Autodesk Inventor part; units mm, degrees
ref_plane "YZ Plane" through (0, 0, 0) normal (1, 0, 0) x (0, 1, 0)
ref_plane "XZ Plane" through (0, 0, 0) normal (0, 1, 0) x (-1, 0, 0)
ref_plane "XY Plane" through (0, 0, 0) normal (0, 0, 1) x (1, 0, 0)
sketch "Sketch1" plane through (0, 0, 0) normal (1, 0, 0) x (0, 1, 0)
  line L0 (-15, 42.5) -> (15, 42.5)
  line L1 (15, 42.5) -> (15, 37.5)
  line L2 (15, 37.5) -> (6.8516, -1.434)
  arc A0 (-6.8516, -1.434) -> (6.8516, -1.434) centre (0, 0) ccw
  line L3 (0, 0) -> (0, 42.5) construction
  line L4 (-15, 42.5) -> (-15, 37.5)
  line L5 (-15, 37.5) -> (-6.8516, -1.434)
  line L6 (-15, 40) -> (15, 40) construction
  arc A1 (4.4, 32.3749) -> (-4.4, 32.3749) centre (0, 30) ccw
  line L7 (-4.4, 32.3749) -> (-4.4, 12.6251)
  line L8 (-4.4, 22.5) -> (4.4, 22.5) construction
  line L9 (4.4, 32.3749) -> (4.4, 12.6251)
  arc A2 (-4.4, 12.6251) -> (4.4, 12.6251) centre (0, 15) ccw
  circle A3 centre (0, 15) radius 15 construction
  line L10 (0, 0) -> (12.9904, 7.5) construction
  line L11 (12.9904, 7.5) -> (25.9808, 15) construction
  line L12 (6, 37.5) -> (-6, 37.5) construction
  line L13 (-6, 37.5) -> (-6, 40) construction
  line L14 (-6, 40) -> (6, 40) construction
  line L15 (6, 40) -> (6, 37.5) construction
  line L16 (6, 37.5) -> (-6, 40) construction
  line L17 (-6, 37.5) -> (6, 40) construction
  arc A4 (4.4, 31.1611) -> (3.6981, 33.3651) centre (2.4943, 31.768) ccw
  arc A5 (-3.6981, 33.3651) -> (-4.4, 31.1611) centre (-2.4943, 31.768) ccw
  arc A6 (3.6981, 11.6349) -> (4.4, 13.8389) centre (2.4943, 13.232) ccw
  arc A7 (-4.4, 13.8389) -> (-3.6981, 11.6349) centre (-2.4943, 13.232) ccw
  circle A8 centre (0, 0) radius 4 construction
  line L18 (6.05, 37.45) -> (-6.05, 37.45)
  line L19 (-6.05, 37.45) -> (-6.05, 40.05)
  line L20 (-6.05, 40.05) -> (6.05, 40.05)
  line L21 (6.05, 40.05) -> (6.05, 37.45)
  line L22 (6.05, 37.45) -> (-6.05, 40.05) construction
  line L23 (-6.05, 37.45) -> (6.05, 40.05) construction
  line L24 (-6.05, 38.75) -> (6.05, 38.75)
  arc A9 (6.05, 40.05) -> (3.05, 40.05) centre (4.55, 40.05) ccw
  arc A10 (3.05, 37.45) -> (6.05, 37.45) centre (4.55, 37.45) ccw
  arc A11 (-3.05, 40.05) -> (-6.05, 40.05) centre (-4.55, 40.05) ccw
  arc A12 (-6.05, 37.45) -> (-3.05, 37.45) centre (-4.55, 37.45) ccw
  circle A13 centre (0, 0) radius 30 construction
  point P0 (-12, 40)
  point P1 (12, 40)
  point P2 (0, 38.75)
  point P3 (-3.6981, 11.6349)
  point P4 (-4.4, 13.8389)
  point P5 (-4.4, 31.1611)
  point P6 (-3.6981, 33.3651)
  point P7 (4.4, 13.8389)
  point P8 (3.6981, 11.6349)
  point P9 (-3.05, 37.45)
  point P10 (-3.05, 40.05)
  point P11 (3.05, 37.45)
  dimension "d0" = 14
  dimension "d1" = 5
  dimension "d3" = 30
  dimension "d4" = 5
  dimension "d5" = 8.8
  dimension "d6" = 15
  dimension "d7" = 60
  dimension "d8" = 15
  dimension "d11" = 24
  dimension "d12" = 12
  dimension "d14" = 2
  dimension "d31" = 8
  dimension "d34" = 1.5
  dimension "d35" = 0.05
  dimension "d36" = 0.05
  dimension "d37" = 5
  dimension "d38" = 2.5
  dimension "d42" = 15
  dimension "d43" = 2.5
extrude "Extrusion1" add sketch "Sketch1" along normal blind 5
hole "Hole1" at (0, -12, 40) at (0, 12, 40) direction (1, 0, 0) diameter 3.5 end through all
hole "Hole2" at (0, 0, 0) direction (1, 0, 0) diameter 8 end through all
equation "\"d36\" = d35"
equation "\"d42\" = d8"
equation "\"d24\" = d31"
properties part number "LegRollSliderFrame" material "Aluminum 7075"
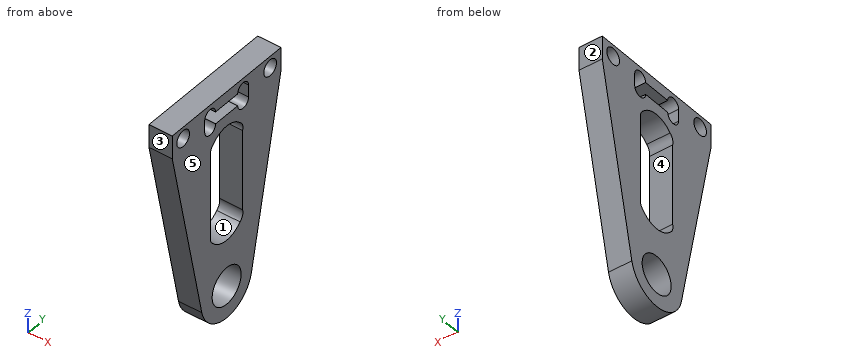
The listing builds one solid part. Answer for the finished solid, in the listing's coordinates (mm). Face numbers are marked on the shaded views. A direction names the side the tool comes from. Give positions to 0.01 mm unless a question says otherwise; leave off trailing zeros. Write each loop counter-clockwise with the first axis right and the second up, starting at its lowest first coordinate (ties: lowest second). Pieces come first, ordered by that corner, then holes.
Item 1: Section D-D, the plane y = -2 is taken. Write down the section's boundary in (x, z), plus the area to 3 significant figures.
Item 2: Section B-B, the plane z = 20.5 is taken. Write down the section's boundary in (x, y), plus the area to 3 significant figures.
Item 3: Find the intervals of material crossed by line 1 along Y through (x, z) = (3.2, 0); line 2 along Y through (x, z) = (3.15, 27); line 3 along Z through (x, y) = (2.25, 2.5), in increasing order.
Item 4: Determine the mould class of the marked faces 1, 2 and 3 for opening direction Y: released by +Y, released by -Y, zero draft, split by the parting line, or undercut.
Item 5: Flat-ended cylindrical pins translate along their axes: P1, Ø3, axis at x = 2, z = 6.5, coming from the +Y side; P2, Ø1.5, axis at x = 3.5, z = 25, coming from the +Y side; P3, Ø2.5, axis at x = 3.5, z = 24.5, coming from the -Y side. Find the tip coordinate at first contact, or state that the pin passes through.
Item 6: Section C-C, the plane y = -5.25 is taken. Write down the section's boundary in (x, z), plus the area to 3 significant figures.
Item 7: Section A-A, the plane x = 2.75 is taken. Write down the section's boundary in (y, z), plus the area to 3 significant figures.
Item 8: Which of the six approach directions +Z, -Z, +X, -X, +Y, -Y give full straight-line access (tool end or side, diameter ignored) to the marked faces 4 and 5?
Completed:
1. outline: (0, -6.71) - (5, -6.71) - (5, -3.46) - (0, -3.46) - close; (0, 3.46) - (5, 3.46) - (5, 10.42) - (0, 10.42) - close; (0, 34.58) - (5, 34.58) - (5, 37.45) - (0, 37.45) - close; (0, 40.05) - (5, 40.05) - (5, 42.5) - (0, 42.5) - close
1. area: 77.6 mm2
2. outline: (0, -11.44) - (5, -11.44) - (5, -4.4) - (0, -4.4) - close; (0, 4.4) - (5, 4.4) - (5, 11.44) - (0, 11.44) - close
2. area: 70.4 mm2
3. line 1: y = -7.15 to -4, 4 to 7.15
3. line 2: y = -12.8 to -4.4, 4.4 to 12.8
3. line 3: z = -6.54 to -3.12, 3.12 to 10.67, 34.33 to 37.45, 40.05 to 42.5
4. face 1: undercut
4. face 2: released by +Y
4. face 3: released by -Y
5. P1: stops at y = 8.83
5. P2: stops at y = 12.54
5. P3: stops at y = -12.54
6. outline: (0, -4.63) - (5, -4.63) - (5, 36.12) - (0, 36.12) - close; (0, 41.38) - (5, 41.38) - (5, 42.5) - (0, 42.5) - close
6. area: 209 mm2
7. outline: (-15, 37.5) - (-6.85, -1.43) arc R7 ccw to (6.85, -1.43) - (15, 37.5) - (15, 42.5) - (-15, 42.5) - close; hole circle Ø3.5 at (-12, 40); hole (-6.05, 37.45) arc R1.5 ccw to (-3.05, 37.45) - (3.05, 37.45) arc R1.5 ccw to (6.05, 37.45) - (6.05, 40.05) arc R1.5 ccw to (3.05, 40.05) - (-3.05, 40.05) arc R1.5 ccw to (-6.05, 40.05) - close; hole (-4.4, 13.84) arc R2 ccw to (-3.7, 11.63) arc R5 ccw to (3.7, 11.63) arc R2 ccw to (4.4, 13.84) - (4.4, 31.16) arc R2 ccw to (3.7, 33.37) arc R5 ccw to (-3.7, 33.37) arc R2 ccw to (-4.4, 31.16) - close; hole circle Ø8 at (0, 0); hole circle Ø3.5 at (12, 40)
7. area: 736 mm2
8. face 4: +X, -X
8. face 5: +Z, -Z, +X, +Y, -Y
